Design review of the part built by this model. Coordinates are the model's own, in mm. A direction names the side the tool comes from. Coordinates: 2 decimals unless noted, no trailing zeros. Loops run counter-clockwise (first coordinate to the right, second up) from the corner with the lowest first, then second, coordinate; pieces in that order, holes last. Notation, with made-up numbers: M 86,67.5 L 92,67.5 A28 ccw 92,100.5 Z; hole C 0.5,20 d10. An arc over 180 degrees is marked long. Put each result on its own line as item: value. Start each with the question number.
(1) Clearance check with flat-ended pins moving along their axes: pin 1 (1.5 mm diameter, centred on y = 2, z = -1.5, fed in from +X) (3 decimals); pin 2 (1 mm diameter, centred on y = 3, z = 2.5, fed in from -X) (3 decimals); pin 3 (0.5 mm diameter, centred on x = -14, y = 1, fed in from -Z). State where each tip first meets the part, or that it passes through.
(2) Take a section at B-B, the plane z = 0. Give the boundary of the cut face in (x, y) (3 decimals), then the cut area to 3 significant figures.
(3) For probe 1 along X at (y, z) = (2.45, 0) (3 decimals); probe 2 along X at (y, z) = (0.3, -1.5) (3 decimals); probe 3 along X at (y, z) = (0.9, 5) (3 decimals), list the stretches that pass through material, from the lowest coordinate up. Write a range as [from, to].
(4) Take a section at C-C, the plane z = -17.5. Give the boundary of the cut face in (x, y) (3 decimals), then the cut area to 3 significant figures.
(5) For faces 5 (the flat face through (-8, 2, -22.225)), 6 (the flat face through (-8, 2, 6.35)), list the 3-axis set-ups (+Z, -Z, +X, -X, +Y, -Y) from which the entire face can be reached by the end or side of a thin tool; tool diameter is ignored.
(6) Take a section at D-D, the plane y = 0.95. Count the separate pieces of the cut face and the enclosed holes in it, then the cut area to 3 significant figures.
(7) The part is to be moulded in two halves that separate along Z. For faces 1 (the cylindrical face through (17.5, 1.61, -4.81)), 2 (the flat face through (3.58, 1.57, -20.84)), 3 (the flat face through (-3.74, 1.61, 8.75)), 4 (the flat face through (12.7, 2, -14)), say which applies: +Z half, -Z half, draft (parallel to the pull), parting line (faces both ways), or undercut.
(8) Take a section at A-A, the plane x = 0. Give the boundary of the cut face in (y, z) (3 decimals).
```python
from build123d import *

# Parameters (mm, degrees)
SKETCH1_R           = 3.175
SKETCH1_W           = 3.175
SKETCH1_H           = 12.7
SKETCH1_H_2         = 6.35
BOSS_EXTRUDE1_DEPTH = 3.175
FILLET1_R           = 1.5875
SKETCH2_R           = 2.38125
CUT_EXTRUDE1_DEPTH  = 46.900442536
FILLET2_R           = 3.175
FILLET4_R           = 0.6
SKETCH3_W           = 59.294957885
SKETCH3_H           = 30.48
CUT_EXTRUDE5_DEPTH  = 46.900442536
FILLET5_R           = 1.5875
CUT_EXTRUDE6_DEPTH  = 34.89972345
SKETCH5_R           = 3.96875
CUT_EXTRUDE7_DEPTH  = 34.89972345
FILLET6_R           = 3.175


with BuildPart() as part:
    # Sketch1 → Boss-Extrude1 (new body)
    with BuildSketch(Plane(origin=(0, 0, 0), x_dir=(1, 0, 0), z_dir=(0, 1, 0))):
        with BuildLine():
            Line((25.4, -12.7), (25.4, -9.525))
            ThreePointArc((25.4, -9.525), (24.935032015, -8.402467985), (23.8125, -7.9375))
            ThreePointArc((23.8125, -7.9375), (22.689967985, -7.472532015), (22.225, -6.35))
            Line((22.225, -6.35), (22.225, 6.35))
            ThreePointArc((22.225, 6.35), (22.689967985, 7.472532015), (23.8125, 7.9375))
            ThreePointArc((23.8125, 7.9375), (24.935032015, 8.402467985), (25.4, 9.525))
            Line((25.4, 9.525), (25.4, 12.7))
            Line((25.4, 12.7), (23.8125, 12.7))
            Line((23.8125, 12.7), (18.25625, 12.7))
            Line((18.25625, 12.7), (11.77006403, 21.29506403))
            ThreePointArc((11.77006403, 21.29506403), (10.740019898, 21.983317516), (9.525, 22.225))
            Line((9.525, 22.225), (6.35, 22.225))
            Line((6.35, 22.225), (0, 19.05))
            Line((0, 19.05), (-6.35, 22.225))
            Line((-6.35, 22.225), (-9.525, 22.225))
            ThreePointArc((-9.525, 22.225), (-10.740019898, 21.983317516), (-11.77006403, 21.29506403))
            Line((-11.77006403, 21.29506403), (-18.25625, 12.7))
            Line((-18.25625, 12.7), (-23.8125, 12.7))
            Line((-23.8125, 12.7), (-25.4, 12.7))
            Line((-25.4, 12.7), (-25.4, 9.525))
            ThreePointArc((-25.4, 9.525), (-24.935032015, 8.402467985), (-23.8125, 7.9375))
            ThreePointArc((-23.8125, 7.9375), (-22.689967985, 7.472532015), (-22.225, 6.35))
            Line((-22.225, 6.35), (-22.225, -6.35))
            ThreePointArc((-22.225, -6.35), (-22.689967985, -7.472532015), (-23.8125, -7.9375))
            ThreePointArc((-23.8125, -7.9375), (-24.935032015, -8.402467985), (-25.4, -9.525))
            Line((-25.4, -9.525), (-25.4, -12.7))
            Line((-25.4, -12.7), (-25.4, -31.75))
            ThreePointArc((-25.4, -31.75), (-20.422679281, -37.949858998), (-13.293464066, -34.430446612))
            Line((-13.293464066, -34.430446612), (-3.175, -12.7))
            Line((-3.175, -12.7), (3.175, -12.7))
            Line((3.175, -12.7), (13.293464066, -34.430446612))
            ThreePointArc((13.293464066, -34.430446612), (20.422679281, -37.949858998), (25.4, -31.75))
            Line((25.4, -31.75), (25.4, -12.7))
        make_face()
        with Locations(Location((-19.05, -31.75, 0), (0, 0, 270))):
            Circle(SKETCH1_R, mode=Mode.SUBTRACT)
        with Locations(Location((19.05, -31.75, 0), (0, 0, 270))):
            Circle(SKETCH1_R, mode=Mode.SUBTRACT)
        with Locations((-7.9375, 0)):
            Rectangle(SKETCH1_W, SKETCH1_H, mode=Mode.SUBTRACT)
        with BuildLine():
            Line((-19.05, -12.7), (-19.05, -22.225))
            ThreePointArc((-19.05, -22.225), (-16.990981078, -22.450211503), (-15.029330082, -23.115196099))
            Line((-15.029330082, -23.115196099), (-10.179646624, -12.7))
            Line((-10.179646624, -12.7), (-19.05, -12.7))
        make_face(mode=Mode.SUBTRACT)
        with BuildLine():
            Line((10.179646624, -12.7), (19.05, -12.7))
            Line((19.05, -12.7), (19.05, -22.225))
            ThreePointArc((19.05, -22.225), (16.990981078, -22.450211503), (15.029330082, -23.115196099))
            Line((15.029330082, -23.115196099), (10.179646624, -12.7))
        make_face(mode=Mode.SUBTRACT)
        with Locations((7.9375, 0)):
            Rectangle(SKETCH1_W, SKETCH1_H, mode=Mode.SUBTRACT)
        with Locations((-7.9375, 15.875)):
            Rectangle(SKETCH1_W, SKETCH1_H_2, mode=Mode.SUBTRACT)
        Polygon((16.267445908, 12.7), (12.7, 12.7), (12.7, 17.427343025), align=None, mode=Mode.SUBTRACT)
        with Locations((7.9375, 15.875)):
            Rectangle(SKETCH1_W, SKETCH1_H_2, mode=Mode.SUBTRACT)
        Polygon((-12.7, 12.7), (-12.7, 17.427343025), (-16.267445908, 12.7), align=None, mode=Mode.SUBTRACT)
    extrude(amount=BOSS_EXTRUDE1_DEPTH)

    # Fillet1
    fillet1_edges = [part.edges().sort_by_distance(p)[0] for p in [
        (3.175, 1.5875, 12.7),
        (-3.175, 1.5875, 12.7),
        (-10.179646624, 1.5875, 12.7),
        (-19.05, 1.5875, 12.7),
        (19.05, 1.5875, 12.7),
        (10.179646624, 1.5875, 12.7),
    ]]
    fillet(fillet1_edges, radius=FILLET1_R)

    # Sketch2 → Cut-Extrude1 (cut, through all)
    with BuildSketch(Plane(origin=(0, 3.175, 0), x_dir=(1, 0, 0), z_dir=(0, 1, 0))):
        with Locations(Location((-17.4625, 7.9375, 0), (0, 0, 270))):
            Circle(SKETCH2_R)
        with Locations(Location((17.4625, 7.9375, 0), (0, 0, 90))):
            Circle(SKETCH2_R)
    extrude(amount=-CUT_EXTRUDE1_DEPTH, mode=Mode.SUBTRACT)

    # Fillet2
    fillet2_edges = [part.edges().sort_by_distance(p)[0] for p in [
        (-6.35, 1.5875, -22.225),
        (0, 1.5875, -19.05),
        (6.35, 1.5875, -22.225),
    ]]
    fillet(fillet2_edges, radius=FILLET2_R)

    # Fillet4
    fillet4_edges = [part.edges().sort_by_distance(p)[0] for p in [
        (18.25625, 1.5875, -12.7),
        (-18.25625, 1.5875, -12.7),
        (16.267445908, 1.5875, -12.7),
        (12.7, 1.5875, -17.427343025),
        (12.7, 1.5875, -12.7),
        (-12.7, 1.5875, -12.7),
        (-12.7, 1.5875, -17.427343025),
        (-16.267445908, 1.5875, -12.7),
    ]]
    fillet(fillet4_edges, radius=FILLET4_R)

    # Sketch3 → Cut-Extrude5 (cut, through all)
    with BuildSketch(Plane(origin=(0, 3.175, 0), x_dir=(1, 0, 0), z_dir=(0, 1, 0))):
        with Locations((-1.965596619, -26.253733592)):
            Rectangle(SKETCH3_W, SKETCH3_H)
    extrude(amount=-CUT_EXTRUDE5_DEPTH, mode=Mode.SUBTRACT)

    # Fillet5
    # the kernel refuses this fillet: 1.5875 mm, written as the material it takes off along each edge
    with BuildSketch(Plane(origin=(25.4, -3.961061605, 11.013733592), x_dir=(0, 0, -1), z_dir=(0, 1, 0))) as fillet5_piece_1:
        with BuildLine():
            CenterArc((1.5875, 1.584424642), FILLET5_R, 180, 86.433035976)
            Line((0, 1.584424642), (-0.03175, 1.584424642))
            Line((-0.03175, 1.584424642), (-0.03175, 0))
            Line((-0.03175, 0), (0, -0.03175))
            ThreePointArc((0, -0.03175), (0.744366796, -0.03175), (1.486758264, -0.031688493))
            Line((1.486758264, -0.031688493), (1.488733592, 0))
        make_face()
    extrude(amount=11.097123211, mode=Mode.SUBTRACT)
    with BuildSketch(Plane(origin=(-25.4, 7.136061605, 11.013733592), x_dir=(1, 0, 0), z_dir=(0, -1, 0))) as fillet5_piece_2:
        with BuildLine():
            CenterArc((1.584424642, -1.5875), FILLET5_R, 90, 86.433035976)
            Line((0, -1.488733592), (-0.031688493, -1.486758264))
            ThreePointArc((-0.031688493, -1.486758264), (-0.03175, -0.744366796), (-0.03175, 0))
            Line((-0.03175, 0), (0, 0.03175))
            Line((0, 0.03175), (1.584424642, 0.03175))
            Line((1.584424642, 0.03175), (1.584424642, 0))
        make_face()
    extrude(amount=11.097123211, mode=Mode.SUBTRACT)

    # Sketch4 → Cut-Extrude6 (cut, through all)
    with BuildSketch(Plane(origin=(0, 3.175, 0), x_dir=(1, 0, 0), z_dir=(0, 1, 0))):
        with BuildLine():
            Line((-15.875, 3.224383204), (-15.875, -6.300616796))
            ThreePointArc((-15.875, -6.300616796), (-17.4625, -7.888116796), (-19.05, -6.300616796))
            Line((-19.05, -6.300616796), (-19.05, 3.224383204))
            ThreePointArc((-19.05, 3.224383204), (-17.4625, 4.811883204), (-15.875, 3.224383204))
        make_face()
        with BuildLine():
            Line((15.875, 3.224383204), (15.875, -6.300616796))
            ThreePointArc((15.875, -6.300616796), (17.4625, -7.888116796), (19.05, -6.300616796))
            Line((19.05, -6.300616796), (19.05, 3.224383204))
            ThreePointArc((19.05, 3.224383204), (17.4625, 4.811883204), (15.875, 3.224383204))
        make_face()
    extrude(amount=-CUT_EXTRUDE6_DEPTH, mode=Mode.SUBTRACT)

    # Sketch5 → Cut-Extrude7 (cut, through all)
    with BuildSketch(Plane(origin=(0, 3.175, 0), x_dir=(1, 0, 0), z_dir=(0, 1, 0))):
        with Locations(Location((0, 0, 0), (0, 0, 270))):
            Circle(SKETCH5_R)
        Polygon((0, -5.506866796), (-6.35, -11.013733592), (6.35, -11.013733592), align=None)
    extrude(amount=-CUT_EXTRUDE7_DEPTH, mode=Mode.SUBTRACT)

    # Fillet6
    fillet6_edges = [part.edges().sort_by_distance(p)[0] for p in [
        (0, 1.5875, 5.506866796),
        (6.35, 1.5875, 11.013733592),
        (-6.35, 1.5875, 11.013733592),
    ]]
    fillet(fillet6_edges, radius=FILLET6_R)


solid = part.part
```
Computed values:
1. pin 1: stops at x = 22.225
1. pin 2: stops at x = -22.225
1. pin 3: stops at z = -18.67
2. outline: M -22.225,0 L -19.05,0 L -19.05,3.175 L -22.225,3.175 Z; M -15.875,0 L -9.525,0 L -9.525,3.175 L -15.875,3.175 Z; M -6.35,0 L -3.969,0 L -3.969,3.175 L -6.35,3.175 Z; M 3.969,0 L 6.35,0 L 6.35,3.175 L 3.969,3.175 Z; M 9.525,0 L 15.875,0 L 15.875,3.175 L 9.525,3.175 Z; M 19.05,0 L 22.225,0 L 22.225,3.175 L 19.05,3.175 Z
2. area: 75.6 mm^2
3. probe 1: x = [-22.225, -19.05], [-15.875, -9.525], [-6.35, -3.969], [3.969, 6.35], [9.525, 15.875], [19.05, 22.225]
3. probe 2: x = [-22.225, -19.05], [-15.875, -9.525], [-6.35, -3.674], [3.674, 6.35], [9.525, 15.875], [19.05, 22.225]
3. probe 3: x = [-22.225, -19.05], [-15.875, -9.525], [-6.35, 6.35], [9.525, 15.875], [19.05, 22.225]
4. outline: M -14.634,0 L -9.525,0 L -9.525,3.175 L -14.634,3.175 Z; M -6.35,0 L 6.35,0 L 6.35,3.175 L -6.35,3.175 Z; M 9.525,0 L 14.634,0 L 14.634,3.175 L 9.525,3.175 Z
4. area: 72.8 mm^2
5. face 5: -Z, +X, -X, +Y, -Y
5. face 6: +Y, -Y
6. separate pieces: 1
6. enclosed holes: 11
6. area: 1,030 mm^2
7. face 1: undercut
7. face 2: -Z half
7. face 3: +Z half
7. face 4: undercut
8. outline: M 0,-19.425 L 3.175,-19.425 L 3.175,-3.969 L 0,-3.969 Z; M 0,3.969 L 3.175,3.969 L 3.175,6.534 L 0,6.534 Z
